The model under review builds one solid part; all positions refer to its coordinate system, in mm. A direction names the side the tool comes from. Coordinates: 2 decimals unless noted, no trailing zeros. Write each loop counter-clockwise with the first axis right and the second up, starting at its lowest first coordinate (ties: lowest second). Pieces come first, ordered by that corner, then holes. Notation, with made-up numbers: M 60,-34 L 89,-34 A21 cw 89,-10 Z; hole C 16.25,-10 d7. An arc over 180 degrees is marked long. Answer as a JSON object with one key per item and string values.
```python
from build123d import *

# Parameters (mm, degrees)
F0_R     = 31.75
F0_R_2   = 10
F1_DEPTH = 304.8
F2_DEPTH = 152.4
F3_DEPTH = 609.6


with BuildPart() as f1:
    # F0 (on Front) → F1 (new body)
    with BuildSketch(Plane.XZ):
        Circle(F0_R)
        Circle(F0_R_2, mode=Mode.SUBTRACT)
        Circle(F0_R_2)
    extrude(amount=-F1_DEPTH)

    # F0 (on Front) → F2 (join)
    with BuildSketch(Plane.XZ):
        Circle(F0_R_2)
    extrude(amount=F2_DEPTH)

    # F3 (add): a face of the model
    f3_faces = [f1.faces().sort_by_distance(p)[0] for p in [
        (0, -152.4, 0),
    ]]
    extrude(f3_faces, amount=-F3_DEPTH)


solid = f1.part
```
(1) For pin 1 Ø10 at (x, z) = (-18, -5.5) entering from +Y; pin 2 Ø10 at (x, z) = (25, 20.5) entering from -Y; pin 3 Ø3 at (y, z) = (312, 9.5) entering from -X, all flat-tipped, find the tip position at first contact; note any pin that passes through.
Results list:
{"pin 1": "y = 304.8", "pin 2": "y = 0", "pin 3": "x = -6"}
(2) Add section D-D on y = 353. Give the boundary of the cut face in (x, z), and give its area (3 significant figures).
Results list:
{"outline": "C 0,0 d20", "area": "314 mm²"}
(3) Add section A-A on z = 0. Give the boundary of the cut face in (x, y), and give its area (3 significant figures).
Results list:
{"outline": "M -31.75,0 L -10,0 L -10,-152.4 L 10,-152.4 L 10,0 L 31.75,0 L 31.75,304.8 L 10,304.8 L 10,457.2 L -10,457.2 L -10,304.8 L -31.75,304.8 Z", "area": "25,500 mm²"}
(4) Add section B-B on x = 0. Give the boundary of the cut face in (y, z), and give its area (3 significant figures).
Results list:
{"outline": "M -152.4,-10 L 0,-10 L 0,-31.75 L 304.8,-31.75 L 304.8,-10 L 457.2,-10 L 457.2,10 L 304.8,10 L 304.8,31.75 L 0,31.75 L 0,10 L -152.4,10 Z", "area": "25,500 mm²"}
(5) For faces 1 (the face through (0, 457.2, 0)), 2 (the face through (-8, 0, 8)), 3 (the face through (-2.17, 379.93, -9.76)), list the 3-axis set-ups (+Z, -Z, +X, -X, +Y, -Y) from which the entire face can be reached by the end or side of a thin tool; tool diameter is ignored.
Results list:
{"face 1": "+Z, -Z, +X, -X, +Y", "face 2": "-Y", "face 3": "+Y"}
(6) Add section C-C on y = 202.5. Give the boundary of the cut face in (x, z), and give its area (3 significant figures).
Results list:
{"outline": "C 0,0 d63.5", "area": "3,170 mm²"}
(7) Wall thickness on line 1 along Y through (x, z) = (-10, 25); line 2 along Z through (x, y) = (1, 273.5); line 3 along Z through (x, y) = (-10, 38): over which ranges is each line inside the solid? List them lowest first. Write a range as from..to.
Results list:
{"line 1": "0..304.8", "line 2": "-31.73..31.73", "line 3": "-30.13..30.13"}
